Design review of the part built by this model. Coordinates are the model's own, in mm. Give positions to 0.01 mm unless a question says otherwise; leave off trailing zeros. Answer in a Markdown table with one row per item. Add a question column.
(1) Consider section A-A on x = 0. Count the separate pieces of the cut face and the enclosed holes in it, then the cut area to 3 significant figures.
(2) Draft analysis for pull direction Z (two halves, no side actions). For faces 1 (the flat face through (-123.825, 6, 410)), 2 (the cylindrical face through (30.284, 28.531, 276.237)), 3 (the cylindrical face through (54.386, -28.619, 362.771)), state which applies: +Z half, -Z half, draft (parallel to the pull), parting line (faces both ways), or undercut.
(3) For line 1 (X direction, y = -27, z = 562) (3 decimals); line 2 (X direction, y = 30, z = 266) (3 decimals); line 3 (X direction, y = 35, z = 680) (3 decimals), list the stretches that pass through material, from the lowest coordinate up.
from build123d import *

# Parameters (mm, degrees)
F0_W     = 12.7
F0_H     = 12.7
F1_DEPTH = 831.85
F2_R     = 31.75
F3_DEPTH = 76.201


with BuildPart() as f1:
    # F0 (on Top) → F1 (new body)
    with BuildSketch(Plane.XY):
        Polygon((-123.825, 44.45), (-136.525, 44.45), (-136.525, -44.45), (-123.825, -44.45), (-123.825, -31.75), (-123.825, -25.4), (-123.825, -12.7), (-123.825, 25.4), (-123.825, 31.75), align=None)
        with Locations((-117.475, 38.1)):
            Rectangle(F0_W, F0_H)
        Polygon((-111.125, 31.75), (-123.825, 31.75), (-123.825, 25.4), (123.825, 25.4), (123.825, 31.75), (111.125, 31.75), align=None)
        with Locations((117.475, 38.1)):
            Rectangle(F0_W, F0_H)
        Polygon((123.825, 31.75), (123.825, 25.4), (123.825, -12.7), (123.825, -25.4), (123.825, -31.75), (123.825, -44.45), (136.525, -44.45), (136.525, 44.45), (123.825, 44.45), align=None)
        with Locations((117.475, -19.05)):
            Rectangle(F0_W, F0_H)
        with Locations((-117.475, -19.05)):
            Rectangle(F0_W, F0_H)
        Polygon((-123.825, -25.4), (-123.825, -31.75), (123.825, -31.75), (123.825, -25.4), (111.125, -25.4), (-111.125, -25.4), align=None)
    extrude(amount=F1_DEPTH)

    # F2 (on face) → F3 (cut, through all)
    with BuildSketch(Plane.XZ.offset(31.75)):
        with Locations((-77.7875, 788.9875)):
            Circle(F2_R)
        with Locations((0, 788.9875)):
            Circle(F2_R)
        with Locations((77.7875, 788.9875)):
            Circle(F2_R)
        with Locations((77.7875, 714.375)):
            Circle(F2_R)
        with Locations((0, 714.375)):
            Circle(F2_R)
        with Locations((-77.7875, 714.375)):
            Circle(F2_R)
        with Locations((-77.7875, 639.7625)):
            Circle(F2_R)
        with Locations((0, 639.7625)):
            Circle(F2_R)
        with Locations((77.7875, 639.7625)):
            Circle(F2_R)
        with Locations((77.7875, 565.15)):
            Circle(F2_R)
        with Locations((0, 565.15)):
            Circle(F2_R)
        with Locations((-77.7875, 565.15)):
            Circle(F2_R)
        with Locations((-77.7875, 490.5375)):
            Circle(F2_R)
        with Locations((0, 490.5375)):
            Circle(F2_R)
        with Locations((77.7875, 490.5375)):
            Circle(F2_R)
        with Locations((77.7875, 415.925)):
            Circle(F2_R)
        with Locations((0, 415.925)):
            Circle(F2_R)
        with Locations((-77.7875, 415.925)):
            Circle(F2_R)
        with Locations((0, 341.3125)):
            Circle(F2_R)
        with Locations((77.7875, 341.3125)):
            Circle(F2_R)
        with Locations((77.7875, 266.7)):
            Circle(F2_R)
        with Locations((0, 266.7)):
            Circle(F2_R)
        with Locations((-77.7875, 266.7)):
            Circle(F2_R)
        with Locations((-77.7875, 341.3125)):
            Circle(F2_R)
        with Locations((-77.7875, 192.0875)):
            Circle(F2_R)
        with Locations((0, 192.0875)):
            Circle(F2_R)
        with Locations((77.7875, 192.0875)):
            Circle(F2_R)
        with Locations((77.7875, 117.475)):
            Circle(F2_R)
        with Locations((0, 117.475)):
            Circle(F2_R)
        with Locations((-77.7875, 117.475)):
            Circle(F2_R)
        with Locations((-77.7875, 42.8625)):
            Circle(F2_R)
        with Locations((0, 42.8625)):
            Circle(F2_R)
        with Locations((77.7875, 42.8625)):
            Circle(F2_R)
    extrude(amount=-F3_DEPTH, mode=Mode.SUBTRACT)


solid = f1.part
Values follow:
| question | item | result |
|---|---|---|
| 1 | separate pieces | 24 |
| 1 | enclosed holes | 0 |
| 1 | area | 1,690 mm2 |
| 2 | face 1 | draft |
| 2 | face 2 | undercut |
| 2 | face 3 | undercut |
| 3 | line 1 | -136.525 to -109.381, -46.194 to -31.593, 31.593 to 46.194, 109.381 to 136.525 |
| 3 | line 2 | -136.525 to -109.53, -46.045 to -31.742, 31.742 to 46.045, 109.53 to 136.525 |
| 3 | line 3 | -136.525 to -111.125, 111.125 to 136.525 |
